```python
from build123d import *

# Parameters (mm, degrees)
F0_W     = 40
F0_H     = 70
F0_R     = 2.5
F1_DEPTH = 4
F2_R     = 2.5
F2_R_2   = 4
F3_DEPTH = 2
F5_DEPTH = 25


with BuildPart() as f1:
    # F0 (on Front) → F1 (new body)
    with BuildSketch(Plane.XZ):
        Rectangle(F0_W, F0_H)
        with Locations((-15, -30)):
            Circle(F0_R, mode=Mode.SUBTRACT)
        with Locations((15, -30)):
            Circle(F0_R, mode=Mode.SUBTRACT)
        with Locations((-15, 30)):
            Circle(F0_R, mode=Mode.SUBTRACT)
        with Locations((15, 30)):
            Circle(F0_R, mode=Mode.SUBTRACT)
    extrude(amount=F1_DEPTH)

    # F2 (on face) → F3 (cut)
    with BuildSketch(Plane.XZ.offset(4)):
        with Locations((-15, 30)):
            Circle(F2_R)
        with Locations((-15, -30)):
            Circle(F2_R)
        with Locations((15, 30)):
            Circle(F2_R)
        with Locations((15, -30)):
            Circle(F2_R)
        with Locations((15, 30)):
            Circle(F2_R_2)
        with Locations((15, 30)):
            Circle(F2_R, mode=Mode.SUBTRACT)
        with Locations((15, -30)):
            Circle(F2_R_2)
        with Locations((15, -30)):
            Circle(F2_R, mode=Mode.SUBTRACT)
        with Locations((-15, -30)):
            Circle(F2_R_2)
        with Locations((-15, -30)):
            Circle(F2_R, mode=Mode.SUBTRACT)
        with Locations((-15, 30)):
            Circle(F2_R_2)
        with Locations((-15, 30)):
            Circle(F2_R, mode=Mode.SUBTRACT)
    extrude(amount=-F3_DEPTH, mode=Mode.SUBTRACT)

    # F4 (on face) → F5 (cut)
    with BuildSketch(Plane.XZ.offset(4)):
        with BuildLine():
            Line((2.921996, -20.153533), (2.921996, -10.71458))
            ThreePointArc((2.921996, -10.71458), (0, 3.692803), (-2.921996, -10.71458))
            Line((-2.921996, -10.71458), (-2.921996, -20.153533))
            ThreePointArc((-2.921996, -20.153533), (0, -22.473871), (2.921996, -20.153533))
        make_face()
    extrude(amount=-F5_DEPTH, mode=Mode.SUBTRACT)


solid = f1.part
```
Read the model definition and answer for the solid it produces. Units are mm, in the model's axes. A direction names the side the tool comes from. Coordinates: 2 decimals unless noted, no trailing zeros. Loops run counter-clockwise (first coordinate to the right, second up) from the corner with the lowest first, then second, coordinate; pieces in that order, holes last.
(1) A flat-ended cylindrical pin translates along its axis: pin 1 Ø4 at (x, z) = (15.5, 29) entering from -Y. Find the tip coordinate at first contact, or state that the pin passes through.
Solution:
pin 1: stops at y = -2
(2) Consider line 1 along Z through (x, y) = (15, -3.1); line 2 along Z through (x, y) = (-15, -1.8); line 3 along X through (y, z) = (-1.45, -19). Determine where each line is inside the solid, lowest interval first.
Solution:
line 1: z = -35 to -34, -26 to 26, 34 to 35
line 2: z = -35 to -32.5, -27.5 to 27.5, 32.5 to 35
line 3: x = -20 to -2.92, 2.92 to 20
(3) The mould has two halves that part along Z. Classify faces 1 (the face through (0, -2, -35)), 2 (the face through (0, -4, 8)), 3 (the face through (13, -2, -32)): released by +Z, released by -Z, zero draft, split by the parting line, or undercut.
Solution:
face 1: released by -Z
face 2: zero draft
face 3: undercut
(4) The part is cut by section A-A (x = 15). Determine the outline of the cut face in (y, z), and give its area (3 significant figures).
Solution:
outline: (-4, -35) - (0, -35) - (0, -32.5) - (-2, -32.5) - (-2, -34) - (-4, -34) - close; (-4, -26) - (-2, -26) - (-2, -27.5) - (0, -27.5) - (0, 27.5) - (-2, 27.5) - (-2, 26) - (-4, 26) - close; (-4, 34) - (-2, 34) - (-2, 32.5) - (0, 32.5) - (0, 35) - (-4, 35) - close
area: 228 mm2
(5) A tool of negligible diameter and unlimited length cuts with its end or side. For faces 4 (the face through (-2.922, -2, -15)), 5 (the face through (17, -2, 32)), 6 (the face through (-20, -2, 0)), from which of +Z, -Z, +X, -X, +Y, -Y can it reach the whole face along a straight path? Write none if from no direction.
Solution:
face 4: +Y, -Y
face 5: -Y
face 6: +Z, -Z, -X, +Y, -Y
(6) The part is cut by section B-B (z = -30). Determine the outline of the cut face in (x, y), and give its area (3 significant figures).
Solution:
outline: (-20, -4) - (-19, -4) - (-19, -2) - (-17.5, -2) - (-17.5, 0) - (-20, 0) - close; (-12.5, -2) - (-11, -2) - (-11, -4) - (11, -4) - (11, -2) - (12.5, -2) - (12.5, 0) - (-12.5, 0) - close; (17.5, -2) - (19, -2) - (19, -4) - (20, -4) - (20, 0) - (17.5, 0) - close
area: 108 mm2
(7) The part is cut by section D-D (x = 0). Determine the outline of the cut face in (y, z), and give its area (3 significant figures).
Solution:
outline: (-4, -35) - (0, -35) - (0, -22.47) - (-4, -22.47) - close; (-4, 3.69) - (0, 3.69) - (0, 35) - (-4, 35) - close
area: 175 mm2
(8) The part is cut by section C-C (y = -2.6). Determine the outline of the cut face in (x, z).
Solution:
outline: (-20, -35) - (20, -35) - (20, 35) - (-20, 35) - close; hole circle Ø8 at (-15, -30); hole circle Ø8 at (-15, 30); hole (-2.92, -20.15) arc R3 ccw to (2.92, -20.15) - (2.92, -10.71) arc R7.5 ccw (long way) to (-2.92, -10.71) - close; hole circle Ø8 at (15, -30); hole circle Ø8 at (15, 30)
